from build123d import *

# Parameters (mm, degrees)
SKETCH1_W           = 40
SKETCH1_H           = 60
BOSS_EXTRUDE1_DEPTH = 28
BOSS_EXTRUDE2_DEPTH = 6.35
FILLET1_R           = 6.35
SKETCH4_W           = 8.790315594
SKETCH4_H           = 9.73
CUT_EXTRUDE1_DEPTH  = 4.6355
SKETCH5_R           = 2
BOSS_EXTRUDE3_DEPTH = 40


with BuildPart() as part:
    # Sketch1 → Boss-Extrude1 (new body)
    with BuildSketch(Plane.XY):
        Rectangle(SKETCH1_W, SKETCH1_H)
    extrude(amount=BOSS_EXTRUDE1_DEPTH)

    # Sketch2 → Boss-Extrude2 (add)
    with BuildSketch(Plane(origin=(0, 0, 0), x_dir=(-1, 0, 0), z_dir=(0, 0, -1))):
        with BuildLine():
            Line((-20, 9.6), (-20, 13.5))
            Line((-20, 13.5), (-26, 13.5))
            Line((-26, 13.5), (-26, 2.5))
            Line((-26, 2.5), (-20, 2.5))
            Line((-20, 2.5), (-20, 6.4))
            Line((-20, 6.4), (-24.038303444, 6.4))
            ThreePointArc((-24.038303444, 6.4), (-25.638303444, 8), (-24.038303444, 9.6))
            Line((-24.038303444, 9.6), (-20, 9.6))
        make_face()
        with BuildLine():
            Line((24.038303444, 6.4), (20, 6.4))
            Line((20, 6.4), (20, 2.5))
            Line((20, 2.5), (26, 2.5))
            Line((26, 2.5), (26, 13.5))
            Line((26, 13.5), (20, 13.5))
            Line((20, 13.5), (20, 9.6))
            Line((20, 9.6), (24.038303444, 9.6))
            ThreePointArc((24.038303444, 9.6), (25.638303444, 8), (24.038303444, 6.4))
        make_face()
    extrude(amount=-BOSS_EXTRUDE2_DEPTH)

    # Fillet1
    fillet1_edges = [part.edges().sort_by_distance(p)[0] for p in [
        (-20, 0, 28),
        (0, -30, 28),
        (20, 0, 28),
        (0, 30, 28),
        (20, -30, 14),
        (-20, -30, 14),
        (-20, 30, 14),
        (20, 30, 14),
    ]]
    fillet(fillet1_edges, radius=FILLET1_R)

    # Sketch4 → Cut-Extrude1 (cut)
    with BuildSketch(Plane.XY.offset(6.35)):
        with Locations((-24.395157797, 8)):
            Rectangle(SKETCH4_W, SKETCH4_H)
        with Locations((24.395157797, 8)):
            Rectangle(SKETCH4_W, SKETCH4_H)
    extrude(amount=-CUT_EXTRUDE1_DEPTH, mode=Mode.SUBTRACT)

    # Sketch5 → Boss-Extrude3 (add, symmetric)
    with BuildSketch(Plane(origin=(0, 0, 0), x_dir=(0, 0, -1), z_dir=(1, 0, 0))):
        with Locations((-14, -16)):
            Circle(SKETCH5_R)
    extrude(amount=BOSS_EXTRUDE3_DEPTH, both=True)


solid = part.part
Build history of the part. All positions in model axes, mm. A direction names the side the tool comes from. Coordinates: 2 decimals unless noted, no trailing zeros. Write each loop counter-clockwise with the first axis right and the second up, starting at its lowest first coordinate (ties: lowest second). Pieces come first, ordered by that corner, then holes.
(1) Cut at C-C on y = -16. List the corners of the cut face in (x, z), and give its area (3 significant figures).
(2) Drill centre lines: line 1 (Y direction, x = -22.5, z = 2.75) (3 decimals); line 2 (X direction, y = -16, z = 9); line 3 (X direction, y = 13, z = 25). Where is each one in solid material? Low to high.
(3) 3-axis set-ups, long thin cutter, end or side, ignore diameter. For faces 1 (the flat face through (22, 6.4, 1)), 2 (the flat face through (-23, 3.135, 4)), 3 (the cylindrical face through (-30, -14, 14)): which of +Z, -Z, +X, -X, +Y, -Y reach the whole face in a straight line?
(4) Cut at A-A on y = 8. List the corners of the cut face in (x, z).
(5) Mould opens along Y. For faces 4 (the cylindrical face through (30, -14, 14)), 5 (the flat face through (0, 30, 11)), 6 (the flat face through (-22, 9.6, 1)), 7 (the flat face through (40, -16, 14)) say: pulls with the +Y half, pulls with the -Y half, needs draft (parallel to the pull), parting line crosses it, or undercut.
(6) Cut at D-D on x = 34.5. List the corners of the cut face in (y, z).
(7) Cut at B-B on z = 14. List the corners of the cut face in (x, y), and give its area (3 significant figures).
(8) Pin check, flat tips, straight feed: pin 1 Ø3.5 at (x, z) = (-23.5, 3) entering from -Y; pin 2 Ø12 at (y, z) = (17.5, 14) entering from -X; pin 3 Ø6 at (x, z) = (-19.5, 8) entering from +Y. Stop position of each tip, or through.
Working result:
1. outline: (-40, 12) - (-20, 12) - (-20, 0) - (20, 0) - (20, 12) - (40, 12) - (40, 16) - (20, 16) - (20, 21.65) arc R6.35 ccw to (13.65, 28) - (-13.65, 28) arc R6.35 ccw to (-20, 21.65) - (-20, 16) - (-40, 16) - close
1. area: 1,260 mm2
2. line 1: y = 2.5 to 3.135, 12.865 to 13.5
2. line 2: x = -20 to 20
2. line 3: x = -19.04 to 19.04
3. face 1: +Z, -Z
3. face 2: +Z, -X
3. face 3: -X
4. outline: (-26, 0) - (-25.64, 0) - (-25.64, 1.71) - (-26, 1.71) - close; (-20, 0) - (20, 0) - (20, 21.65) arc R6.35 ccw to (13.65, 28) - (-13.65, 28) arc R6.35 ccw to (-20, 21.65) - close; (25.64, 0) - (26, 0) - (26, 1.71) - (25.64, 1.71) - close
5. face 4: parting line crosses it
5. face 5: pulls with the +Y half
5. face 6: undercut
5. face 7: needs draft
6. outline: circle Ø4 at (-16, 14)
7. outline: (-40, -18) - (-20, -18) - (-20, -23.65) arc R6.35 ccw to (-13.65, -30) - (13.65, -30) arc R6.35 ccw to (20, -23.65) - (20, -18) - (40, -18) - (40, -14) - (20, -14) - (20, 23.65) arc R6.35 ccw to (13.65, 30) - (-13.65, 30) arc R6.35 ccw to (-20, 23.65) - (-20, -14) - (-40, -14) - close
7. area: 2,530 mm2
8. pin 1: stops at y = 2.5
8. pin 2: stops at x = -20
8. pin 3: stops at y = 29.32
